Can you work these out from the drawing? Everything is in mm from the part's minimum corner. A direction names the side the tool comes from. Round coordinates to 2 decimals unless told otherwise and drop trailing zeros. Order: outer loops, then holes, each group sorted by start corner. A loop starts at its lowest first (then second) coordinate and runs counter-clockwise, first axis right, second up. Notation, with made-up numbers: (-3.75, 24) -> (53.25, 24) arc R34 cw to (53.25, 62) -> close; hole circle Ø2 at (29, 45.25). An arc over 180 degrees is marked (long way). One line per item, written item: value.
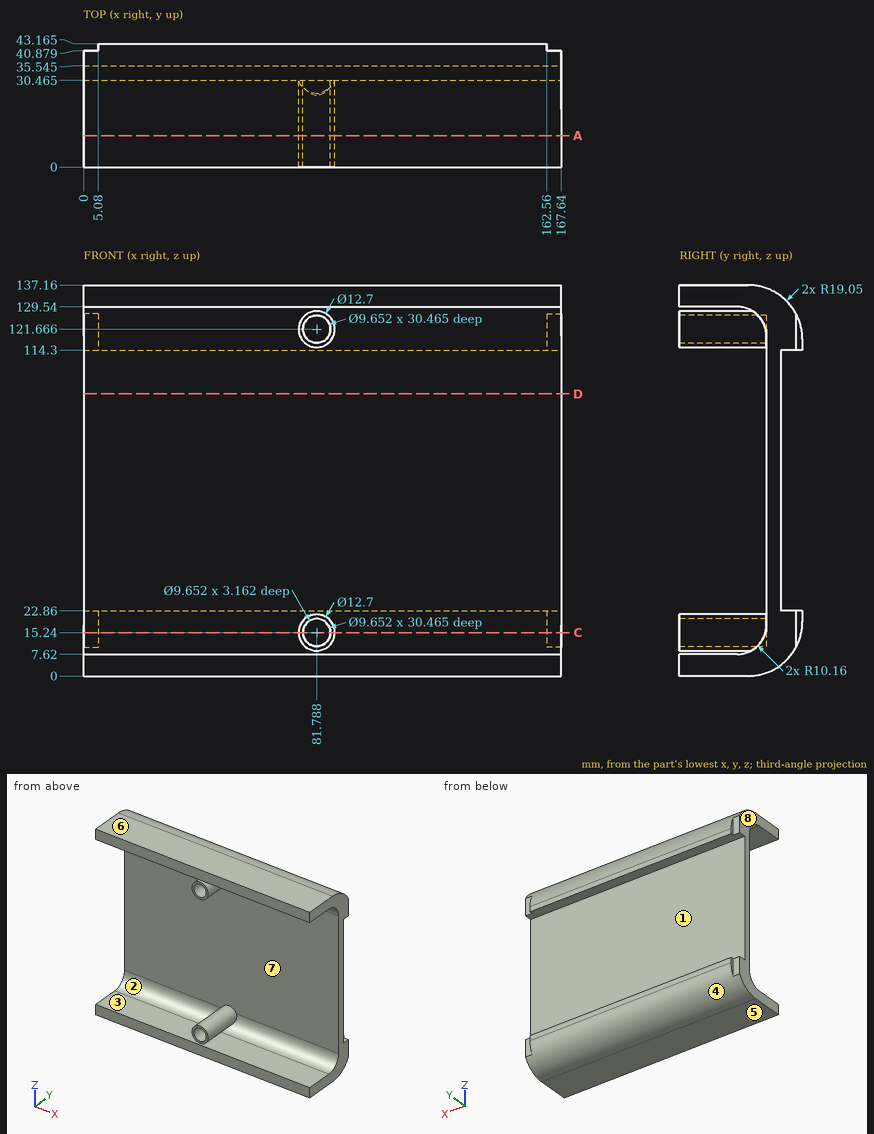
Q1. I need wall thicknesses on line 1 along X through (y, z) = (24, 15.24); line 2 along Z through (x, y) = (7.5, 7.5); line 3 along Y through (x, z) = (29, 92.5) (1 decimal). Which ranges of each line are inside material? Lowest first, please.
Answers:
line 1: 75.44 to 76.96, 86.61 to 88.14
line 2: 0 to 7.62, 129.54 to 137.16
line 3: 30.5 to 35.5
Q2. For P1, Ø3, axis at x = 149.5, z = 119, coming from the -Y side; P2, Ø5, axis at x = 62, z = 122, coming from the +Y side; P3, Ø2, axis at x = 17.5, y = 30.5, coming from the -Z side; P4, Ø7.5, axis at x = 81.788, z = 15.24, coming from the +Y side (1 decimal), each with a flat end and sliding along its axis, tell me the tip position at first contact or that it passes through.
Answers:
P1: y = 30.4
P2: y = 43.11
P3: z = 0.78
P4: y = 43.2
Q3. I want a section at C-C on z = 15.24. Write out the boundary of the cut face in (x, y) (1 decimal), then the cut area to 3 significant figures.
Answers:
outline: (0, 30.1) -> (75.4, 30.1) -> (75.4, 0) -> (77, 0) -> (77, 30.5) -> (86.6, 30.5) -> (86.6, 0) -> (88.1, 0) -> (88.1, 30.1) -> (167.6, 30.1) -> (167.6, 40.9) -> (162.6, 40.9) -> (162.6, 42.8) -> (5.1, 42.8) -> (5.1, 40.9) -> (0, 40.9) -> close
area: 2,190 mm2
Q4. Which directions (+Z, -Z, +X, -X, +Y, -Y) give clear straight access to the entire face, cutting with the end or side of a thin tool? Please do the marked faces 1, 2, 3 and 4.
Answers:
face 1: +X, -X, +Y
face 2: -Y
face 3: +X, -X, -Y
face 4: -Z, +X, -X, +Y
Q5. I want a section at A-A on y = 11. Write out the boundary of the cut face in (x, z).
Answers:
outline: (0, 0) -> (167.64, 0) -> (167.64, 7.62) -> (0, 7.62) -> close; (0, 129.54) -> (167.64, 129.54) -> (167.64, 137.16) -> (0, 137.16) -> close; circle Ø12.7 at (81.79, 15.24); circle Ø12.7 at (81.79, 121.67); hole circle Ø9.65 at (81.79, 15.24); hole circle Ø9.65 at (81.79, 121.67)
Q6. If we mould it in two halves opening along Z, with no side actions, what happens to the marked faces 5, 6, 7 and 8? For each: pulls with the +Z half, pulls with the -Z half, needs draft (parallel to the pull), parting line crosses it, or undercut.
Answers:
face 5: pulls with the -Z half
face 6: pulls with the +Z half
face 7: undercut
face 8: needs draft
Q7. I want a section at D-D on z = 99. Write out the boundary of the cut face in (x, y) (1 decimal).
Answers:
outline: (0, 30.5) -> (167.6, 30.5) -> (167.6, 35.5) -> (0, 35.5) -> close
